from build123d import *

# Parameters (mm, degrees)
SKETCH2_W           = 6
SKETCH2_H           = 10
BOSS_EXTRUDE1_DEPTH = 42
SKETCH3_R           = 11
BOSS_EXTRUDE2_DEPTH = 10
SKETCH4_R           = 7.5
CUT_EXTRUDE1_DEPTH  = 2
SKETCH6_R           = 3
CUT_EXTRUDE2_DEPTH  = 13
FILLET1_R           = 2
CUT_EXTRUDE3_REACH  = 46.553
SKETCH7_R           = 1.5


with BuildPart() as part:
    # Sketch2 → Boss-Extrude1 (new body)
    with BuildSketch(Plane(origin=(0, 0, 0), x_dir=(0, 0, -1), z_dir=(1, 0, 0))):
        Rectangle(SKETCH2_W, SKETCH2_H)
    extrude(amount=BOSS_EXTRUDE1_DEPTH)

    # Sketch3 → Boss-Extrude2 (add)
    with BuildSketch(Plane(origin=(0, 5, 0), x_dir=(1, 0, 0), z_dir=(0, 1, 0))):
        with Locations((21, 0)):
            Circle(SKETCH3_R)
    extrude(amount=-BOSS_EXTRUDE2_DEPTH)

    # Sketch4 → Cut-Extrude1 (cut)
    with BuildSketch(Plane(origin=(0, -5, 0), x_dir=(-1, 0, 0), z_dir=(0, -1, 0))):
        with Locations(Location((-21, 0, 0), (0, 0, 90))):
            Circle(SKETCH4_R)
    extrude(amount=-CUT_EXTRUDE1_DEPTH, mode=Mode.SUBTRACT)

    # Sketch5 → Cut-Revolve1 (revolve, cut)
    with BuildSketch(Plane(origin=(0, 0, 0), x_dir=(-1, 0, 0), z_dir=(0, 0, -1)), mode=Mode.PRIVATE) as cut_revolve1_sk:
        Polygon((-21, -3), (-28.5, -3), (-23.5, 2), (-21, 2), align=None)
    revolve(cut_revolve1_sk.sketch.rotate(Axis((21, 2, 0), (0, -1, 0)), 270), axis=Axis((21, 2, 0), (0, -1, 0)), mode=Mode.SUBTRACT)

    # Sketch6 → Cut-Extrude2 (cut)
    with BuildSketch(Plane.XZ.offset(-2)):
        with Locations(Location((21, 0, 0), (0, 0, 270))):
            Circle(SKETCH6_R)
    extrude(amount=-CUT_EXTRUDE2_DEPTH, mode=Mode.SUBTRACT)

    # Fillet1
    fillet1_edges = [part.edges().sort_by_distance(p)[0] for p in [
        (21, -5, 7.5),
    ]]
    fillet(fillet1_edges, radius=FILLET1_R - 0.0001)  # a hair under: the kernel refuses the full size

    # Sketch7 → Cut-Extrude3 (cut, up to next)
    with BuildSketch(Plane.XZ.offset(5), mode=Mode.PRIVATE) as cut_extrude3_sk1:
        with Locations(Location((5, 0, 0), (0, 0, 270))):
            Circle(SKETCH7_R)
    cut_extrude3_tool1 = extrude(cut_extrude3_sk1.sketch, amount=-CUT_EXTRUDE3_REACH, mode=Mode.PRIVATE) & part.part
    # Sketch7 → Cut-Extrude3 (cut, up to next)
    with BuildSketch(Plane.XZ.offset(5), mode=Mode.PRIVATE) as cut_extrude3_sk2:
        with Locations(Location((37, 0, 0), (0, 0, 270))):
            Circle(SKETCH7_R)
    cut_extrude3_tool2 = extrude(cut_extrude3_sk2.sketch, amount=-CUT_EXTRUDE3_REACH, mode=Mode.PRIVATE) & part.part
    add(cut_extrude3_tool1.solids().sort_by_distance((5, -5, 0))[0], mode=Mode.SUBTRACT)
    add(cut_extrude3_tool2.solids().sort_by_distance((37, -5, 0))[0], mode=Mode.SUBTRACT)


solid = part.part
Model file for the job. Use its own axes, mm. A direction names the side the tool comes from. Round coordinates to 2 decimals unless told otherwise and drop trailing zeros. Order: outer loops, then holes, each group sorted by start corner. A loop starts at its lowest first (then second) coordinate and runs counter-clockwise, first axis right, second up.
(1) Band-saw the part on A-A (x = 5). List the corners of the cut face in (y, z).
(2) 3-axis set-ups, long thin cutter, end or side, ignore diameter. For faces 5 (the face through (37, 0, 3)), 6 (the face through (37, 0, -3)), 7 (the face through (21.9, 3.48, -2.86)), 8 (the face through (5, 0, 3)), 9 (the face through (5, 0, -3)): which of +Z, -Z, +X, -X, +Y, -Y reach the whole face in a straight line?
(3) Pull direction X, two halves, no side cores. Call faces 1 (the face through (5.45, -0.07, -1.43)), 2 (the face through (23, 2, 2)), 3 (the face through (21, 0, 11)), 4 (the face through (0, 0, 0)): released by +X, released by -X, zero draft, split by the parting line, or undercut.
(4) Pin check, flat tips, straight feed: pin 1 (1.5 mm diameter, centred on x = 36.5, y = 1.5, fed in from +Z); pin 2 (3 mm diameter, centred on x = 37.5, y = 0.5, fed in from -Z); pin 3 (5 mm diameter, centred on x = 11, y = 2.5, fed in from -Z). Stop position of each tip, or through.
(5) Drill centre lines: line 1 (X direction, y = -3, z = 0); line 2 (X direction, y = -1, z = 0); line 3 (Z direction, x = 37.5, y = -2). Where is each one in solid material? Low to high.
(6) Band-saw the part on B-B (z = 0). Give the number of separate pieces and of enclosed holes in the cut face, then the cut area to 3 significant figures.
(7) Band-saw the part on C-C (y = 3). List the corners of the cut face in (x, z).
Verdict:
1. outline: (-5, -3) - (5, -3) - (5, -1.5) - (-5, -1.5) - close; (-5, 1.5) - (5, 1.5) - (5, 3) - (-5, 3) - close
2. face 5: +Z, +X, +Y, -Y
2. face 6: -Z, +X, +Y, -Y
2. face 7: +Y
2. face 8: +Z, -X, +Y, -Y
2. face 9: -Z, -X, +Y, -Y
3. face 1: undercut
3. face 2: undercut
3. face 3: split by the parting line
3. face 4: released by -X
4. pin 1: stops at z = 3
4. pin 2: stops at z = -3
4. pin 3: stops at z = -8.05
5. line 1: x = 0 to 3.5, 6.5 to 13.5, 28.5 to 35.5, 38.5 to 42
5. line 2: x = 0 to 3.5, 6.5 to 15.5, 26.5 to 35.5, 38.5 to 42
5. line 3: z = -3 to -1.41, 1.41 to 3
6. separate pieces: 4
6. enclosed holes: 0
6. area: 260 mm2
7. outline: (0, -3) - (10.42, -3) arc R11 ccw to (31.58, -3) - (42, -3) - (42, 3) - (31.58, 3) arc R11 ccw to (10.42, 3) - (0, 3) - close; hole circle Ø3 at (5, 0); hole circle Ø6 at (21, 0); hole circle Ø3 at (37, 0)
